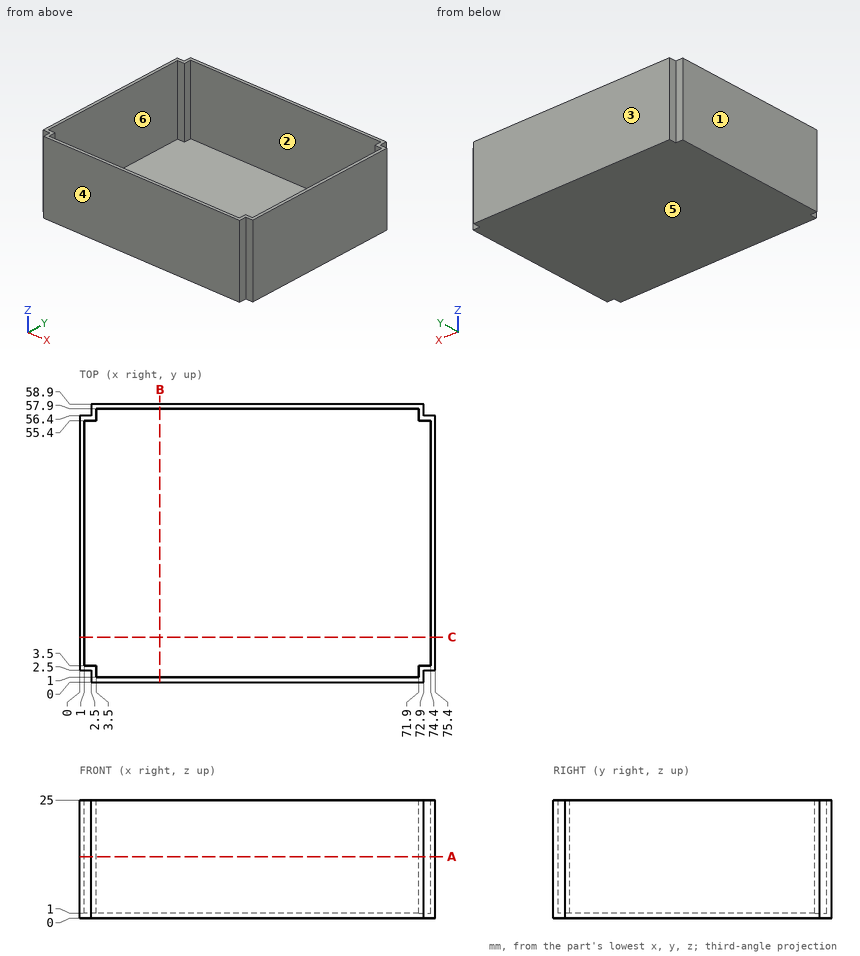
Input: dimensioned drawing with shaded views. Units: mm. Origin: part minimum x, y, z. A direction names the side the tool comes from. Coordinates: 2 decimals unless noted, no trailing zeros. Loops run counter-clockwise (first coordinate to the right, second up) from the corner with the lowest first, then second, coordinate; pieces in that order, holes last. Notation, with made-up numbers: M 64,-30.5 L 92,-30.5 A7 cw 92,-19.5 Z; hole C -32,37 d9. An arc over 180 degrees is marked long. One line per item, written item: value.
(1) Section A-A (z = 13). Output: boundary loops of the cut face in (x, y).
Filled in:
outline: M 0,2.5 L 2.5,2.5 L 2.5,0 L 72.9,0 L 72.9,2.5 L 75.4,2.5 L 75.4,56.4 L 72.9,56.4 L 72.9,58.9 L 2.5,58.9 L 2.5,56.4 L 0,56.4 Z; hole M 1,3.5 L 3.5,3.5 L 3.5,1 L 71.9,1 L 71.9,3.5 L 74.4,3.5 L 74.4,55.4 L 71.9,55.4 L 71.9,57.9 L 3.5,57.9 L 3.5,55.4 L 1,55.4 Z
(2) Section B-B (x = 17). Output: boundary loops of the cut face in (y, z).
Filled in:
outline: M 0,0 L 58.9,0 L 58.9,25 L 57.9,25 L 57.9,1 L 1,1 L 1,25 L 0,25 Z
(3) Reachability of the marked faces 1 and 2 from +Z, -Z, +X, -X, +Y, -Y: full face, straight path, thin tool, end or side. Return the list, or none.
Filled in:
face 1: +Z, -Z, -X, +Y, -Y
face 2: +Z
(4) Pin query (flat end, axial travel): pin 1 (2 mm diameter, centred on y = 57.5, z = 14, fed in from +X); pin 2 (0.8 mm diameter, centred on x = 2.5, z = 16, fed in from -Y); pin 3 (0.8 mm diameter, centred on y = 1.5, z = 12.5, fed in from -X); pin 4 (0.8 mm diameter, centred on x = 2, z = 11, fed in from +Y). Return the tip coordinate at first contact, or that it passes through.
Filled in:
pin 1: x = 72.9
pin 2: y = 0
pin 3: x = 2.5
pin 4: y = 56.4
(5) Pull-direction query (Y, two-part tool) for the marked faces 3, 4, 5 and 6; classes: +Y half, -Y half, draft (parallel to the pull), parting line (faces both ways), or undercut.
Filled in:
face 3: +Y half
face 4: -Y half
face 5: draft
face 6: undercut
(6) Line query: line 1 along Y through (x, z) = (47.5, 23); line 2 along X through (y, z) = (36.5, 15.25); line 3 along Z through (x, y) = (28, 37). Output: solid intervals per line, ascending. Write a range as from..to.
Filled in:
line 1: 0..1, 57.9..58.9
line 2: 0..1, 74.4..75.4
line 3: 0..1
(7) Section C-C (y = 9.5). Output: boundary loops of the cut face in (x, z), and give its area (3 significant figures).
Filled in:
outline: M 0,0 L 75.4,0 L 75.4,25 L 74.4,25 L 74.4,1 L 1,1 L 1,25 L 0,25 Z
area: 123 mm^2
